from build123d import *

# Parameters (mm, degrees)
SKETCH1_R           = 10.2
BOSS_EXTRUDE1_DEPTH = 3
CHAMFER1_SIZE       = 0.5


with BuildPart() as part:
    # Sketch1 → Boss-Extrude1 (new body)
    with BuildSketch(Plane.XY):
        Circle(SKETCH1_R)
        with BuildLine():
            Line((-2.133072901, 2.9), (2.133072901, 2.9))
            ThreePointArc((2.133072901, 2.9), (3.6, 0), (2.133072901, -2.9))
            Line((2.133072901, -2.9), (-2.133072901, -2.9))
            ThreePointArc((-2.133072901, -2.9), (-3.6, 0), (-2.133072901, 2.9))
        make_face(mode=Mode.SUBTRACT)
    extrude(amount=BOSS_EXTRUDE1_DEPTH)

    # Chamfer1
    chamfer1_edges = [part.edges().sort_by_distance(p)[0] for p in [
        (3.6, 0, 3),
        (0, 2.9, 3),
        (-10.2, 0, 0),
        (-10.2, 0, 3),
        (-3.6, 0, 0),
        (0, -2.9, 0),
        (3.6, 0, 0),
        (0, 2.9, 0),
        (-3.6, 0, 3),
        (0, -2.9, 3),
    ]]
    chamfer(chamfer1_edges, length=CHAMFER1_SIZE)


solid = part.part
Source: CAD feature listing. Evaluate the final solid. Frame: model axes, mm. A direction names the side the tool comes from. Coordinates: 2 decimals unless noted, no trailing zeros. Write each loop counter-clockwise with the first axis right and the second up, starting at its lowest first coordinate (ties: lowest second). Pieces come first, ordered by that corner, then holes. Notation, with made-up numbers: M 56,22 L 93,22 A6 cw 93,31 Z; hole C 39,8 d8. An arc over 180 degrees is marked long. Use a Markdown table: item, result.
1) Ray query, L1, parallel to X at y = 2.5, z = 0.85; L2, parallel to Y at x = -2, z = 1.35; L3, parallel to X at y = 0.75, z = 1.4. Return the intervals inside material, ascending.
Conclusion:
| item | result |
|---|---|
| L1 | x = -9.89 to -2.59, 2.59 to 9.89 |
| L2 | y = -10 to -2.9, 2.9 to 10 |
| L3 | x = -10.17 to -3.52, 3.52 to 10.17 |
2) Section A-A, the plane x = 0. Output: boundary loops of the cut face in (y, z), then the cut area to 3 significant figures.
Conclusion:
| item | result |
|---|---|
| outline | M -10.2,0.5 L -9.7,0 L -3.4,0 L -2.9,0.5 L -2.9,2.5 L -3.4,3 L -9.7,3 L -10.2,2.5 Z; M 2.9,0.5 L 3.4,0 L 9.7,0 L 10.2,0.5 L 10.2,2.5 L 9.7,3 L 3.4,3 L 2.9,2.5 Z |
| area | 42.8 mm^2 |
3) Section C-C, the plane z = 1.55. Output: boundary loops of the cut face in (x, y), then the cut area to 3 significant figures.
Conclusion:
| item | result |
|---|---|
| outline | C 0,0 d20.4; hole M -2.13,-2.9 L 2.13,-2.9 A3.6 ccw 2.13,2.9 L -2.13,2.9 A3.6 ccw Z |
| area | 290 mm^2 |
4) Mould query, pull axis X, two halves, no side actions, for faces 1 (the cylindrical face through (4.707, -9.049, 1.486)), 2 (the conical face through (-3.74, -0.05, 2.64)), 3 (the conical face through (3.74, 0.05, 2.64)), 4 (the flat face through (0, -4, 0)). Classes: pulls with the +X half, pulls with the -X half, needs draft (parallel to the pull), parting line crosses it, or undercut.
Conclusion:
| item | result |
|---|---|
| face 1 | parting line crosses it |
| face 2 | undercut |
| face 3 | undercut |
| face 4 | needs draft |
5) Section D-D, the plane z = 0.25. Output: boundary loops of the cut face in (x, y), then the cut area to 3 significant figures.
Conclusion:
| item | result |
|---|---|
| outline | C 0,0 d19.9; hole M -2.21,-3.15 L 2.21,-3.15 A3.85 ccw 2.21,3.15 L -2.21,3.15 A3.85 ccw Z |
| area | 269 mm^2 |
6) First-contact query: pin 1 Ø8 at (x, y) = (4, 6.5) entering from -Z. Flat tip, straight axial feed; report the tip coordinate or a pass-through.
Conclusion:
| item | result |
|---|---|
| pin 1 | stops at z = 0 |
7) Reachability of faces 5 (the cylindrical face through (-3.6, 0, 1.5)), 6 (the conical face through (-3.74, -0.05, 0.36)), 7 (the flat face through (0, -4, 3)) from +Z, -Z, +X, -X, +Y, -Y: full face, straight path, thin tool, end or side. Return the list, or none.
Conclusion:
| item | result |
|---|---|
| face 5 | +Z, -Z |
| face 6 | -Z |
| face 7 | +Z, +X, -X, +Y, -Y |
8) Section B-B, the plane y = 0. Output: boundary loops of the cut face in (x, z).
Conclusion:
| item | result |
|---|---|
| outline | M -10.2,0.5 L -9.7,0 L -4.1,0 L -3.6,0.5 L -3.6,2.5 L -4.1,3 L -9.7,3 L -10.2,2.5 Z; M 3.6,0.5 L 4.1,0 L 9.7,0 L 10.2,0.5 L 10.2,2.5 L 9.7,3 L 4.1,3 L 3.6,2.5 Z |
